Verification items for this drawing (mm, ordinates from the low corner). Give positions to 0.01 mm unless a question says otherwise; leave off trailing zeros. Loops run counter-clockwise (first coordinate to the right, second up) from the corner with the lowest first, then second, coordinate; pieces in that order, holes last. Notation, with made-up numbers: (88, 88) -> (131, 88) arc R11 cw to (131, 107) -> close; hole circle Ø8 at (69.25, 89.25). An arc over 180 degrees is marked (long way). Answer in a Markdown table with one row per item. Add a question column.
Q1. Material ranges on probe 1 along X at (y, z) = (1.4, 20.05); probe 2 along X at (y, z) = (1.25, 19); probe 3 along X at (y, z) = (0.7, 32.5), recorded low to high.
Q2. Section check C-C on x = 28.05. Enter the section's corners in (y, z).
Q3. Section check A-A on z = 20.05. Enter the section's corners in (x, y), and give its area (3 significant figures).
Q4. Section check D-D on x = 34. Enter the section's corners in (y, z).
Q5. Section check B-B on y = 0.65. Give the number of separate pieces and of enclosed holes in the cut face, and give its area (3 significant figures).
Q6. Gauge pin test, flat ends, axial feed: P1, Ø1, axis at y = 0.5, z = 18.5, coming from the -X side; P2, Ø1, axis at y = 1, z = 7, coming from the +X side; P3, Ø1, axis at x = 6, y = 0.5, coming from the +Z side. Record the tip position at first contact, or that the pin passes through.
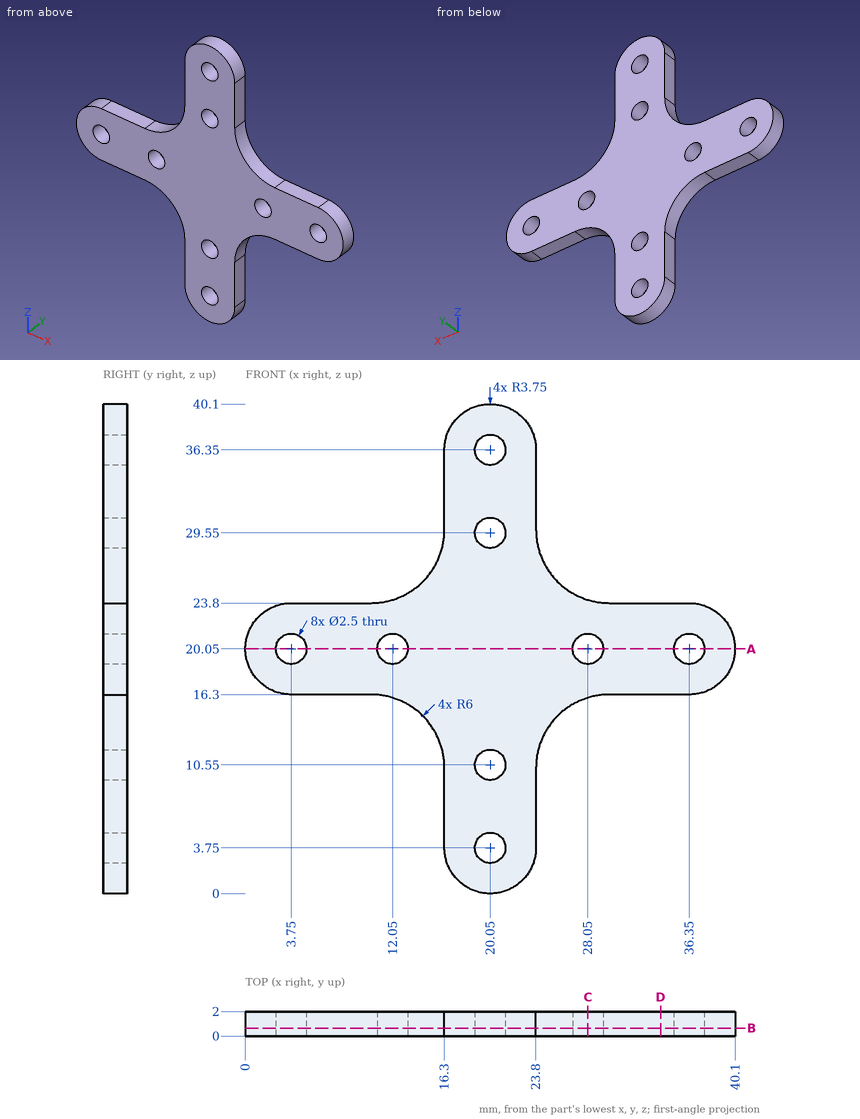
Taken from the geometry:
| question | item | result |
|---|---|---|
| 1 | probe 1 | x = 0 to 2.5, 5 to 10.8, 13.3 to 26.8, 29.3 to 35.1, 37.6 to 40.1 |
| 1 | probe 2 | x = 0.15 to 3.07, 4.43 to 11.37, 12.73 to 27.37, 28.73 to 35.67, 37.03 to 39.95 |
| 1 | probe 3 | x = 16.3 to 23.8 |
| 2 | outline | (0, 16.04) -> (2, 16.04) -> (2, 18.8) -> (0, 18.8) -> close; (0, 21.3) -> (2, 21.3) -> (2, 24.06) -> (0, 24.06) -> close |
| 3 | outline | (0, 0) -> (2.5, 0) -> (2.5, 2) -> (0, 2) -> close; (5, 0) -> (10.8, 0) -> (10.8, 2) -> (5, 2) -> close; (13.3, 0) -> (26.8, 0) -> (26.8, 2) -> (13.3, 2) -> close; (29.3, 0) -> (35.1, 0) -> (35.1, 2) -> (29.3, 2) -> close; (37.6, 0) -> (40.1, 0) -> (40.1, 2) -> (37.6, 2) -> close |
| 3 | area | 60.2 mm² |
| 4 | outline | (0, 16.3) -> (2, 16.3) -> (2, 23.8) -> (0, 23.8) -> close |
| 5 | separate pieces | 1 |
| 5 | enclosed holes | 8 |
| 5 | area | 513 mm² |
| 6 | P1 | stops at x = 0.15 |
| 6 | P2 | stops at x = 23.8 |
| 6 | P3 | stops at z = 23.8 |
